```python
from build123d import *

# Parameters (mm, degrees)
SKETCH1_W           = 50
SKETCH1_H           = 200
BOSS_EXTRUDE1_DEPTH = 15
BOSS_EXTRUDE2_DEPTH = 20
BOSS_EXTRUDE3_DEPTH = 15


with BuildPart() as part:
    # Sketch1 → Boss-Extrude1 (new body)
    with BuildSketch(Plane(origin=(0, 0, 0), x_dir=(1, 0, 0), z_dir=(0, 1, 0))):
        Rectangle(SKETCH1_W, SKETCH1_H)
    extrude(amount=BOSS_EXTRUDE1_DEPTH)

    # Sketch2 → Boss-Extrude2 (add)
    with BuildSketch(Plane(origin=(0, 0, -30), x_dir=(-1, 0, 0), z_dir=(0, 0, -1))):
        with BuildLine():
            Line((25, 15), (25, 265))
            Line((25, 265), (-225, 265))
            Line((-225, 265), (-225, 215))
            ThreePointArc((-225, 215), (-82.144079422, 157.855920578), (-25, 15))
            Line((-25, 15), (25, 15))
        make_face()
        with BuildLine():
            Line((-25, 228.25), (-175, 228.25))
            ThreePointArc((-175, 228.25), (-186.75, 240), (-175, 251.75))
            Line((-175, 251.75), (-25, 251.75))
            ThreePointArc((-25, 251.75), (-13.25, 240), (-25, 228.25))
        make_face(mode=Mode.SUBTRACT)
    extrude(amount=BOSS_EXTRUDE2_DEPTH)

    # Sketch4 → Boss-Extrude3 (add)
    with BuildSketch(Plane.ZY.offset(7.5)):
        Polygon((-30, 115), (70, 15), (-30, 15), align=None)
    extrude(amount=-BOSS_EXTRUDE3_DEPTH)


solid = part.part
```
The model under review builds one solid part; all positions refer to its coordinate system, in mm. A direction names the side the tool comes from. Round coordinates to 2 decimals unless told otherwise and drop trailing zeros. Loops run counter-clockwise (first coordinate to the right, second up) from the corner with the lowest first, then second, coordinate; pieces in that order, holes last.
Item 1: Take a section at C-C (z = 38). Write out the cut boundary in (x, y).
Determined:
outline: (-25, 0) - (25, 0) - (25, 15) - (7.5, 15) - (7.5, 47) - (-7.5, 47) - (-7.5, 15) - (-25, 15) - close
Item 2: Clearance check with flat-ended pins moving along their axes: pin 1 Ø10 at (x, y) = (58.5, 198) entering from -Z; pin 2 Ø12 at (x, y) = (57, 127.5) entering from +Z; pin 3 Ø15 at (x, z) = (-12.5, 51.5) entering from +Y. State where each tip first meets the part, or that it passes through.
Determined:
pin 1: stops at z = -50
pin 2: stops at z = -30
pin 3: stops at y = 39.09
Item 3: For faces 4 (the face through (-11, 15, 34)), 5 (the face through (7.5, 43, -2)), 6 (the face through (74, 170, -50)), 7 (the face through (13.253, 240.258, -39.86)), list the 3-axis set-ups (+Z, -Z, +X, -X, +Y, -Y) from which the entire face can be reached by the end or side of a thin tool; tool diameter is ignored.
Determined:
face 4: +Z, +Y
face 5: +Z, +X, +Y
face 6: -Z, +X, -X, +Y
face 7: +Z, -Z
Item 4: Take a section at A-A (y = 240). Write out the cut boundary in (x, z), then the cut area to 3 significant figures.
Determined:
outline: (-25, -50) - (13.25, -50) - (13.25, -30) - (-25, -30) - close; (186.75, -50) - (225, -50) - (225, -30) - (186.75, -30) - close
area: 1,530 mm2
Item 5: Take a section at B-B (x = 126.5). Write out the cut boundary in (y, z).
Determined:
outline: (191.09, -50) - (228.25, -50) - (228.25, -30) - (191.09, -30) - close; (251.75, -50) - (265, -50) - (265, -30) - (251.75, -30) - close
Item 6: For line 1 (Z direction, x = 5.5, y = 137.5); line 2 (Y direction, x = 93.5, z = -37.5); line 3 (X direction, y = 31, z = 13.5), list the stretches that pass through material, from the lowest coordinate up.
Determined:
line 1: z = -50 to -30
line 2: y = 168.35 to 228.25, 251.75 to 265
line 3: x = -7.5 to 7.5
Item 7: Mouldability with a two-part tool opening along Y and no side actions: class faces 1 (the face through (0, 15, -75)), 2 (the face through (225, 240, -40)), 3 (the face through (101, 251.75, -40)) as released by +Y, released by -Y, zero draft, split by the parting line, or undercut.
Determined:
face 1: released by +Y
face 2: zero draft
face 3: undercut
Item 8: Take a section at D-D (y = 57). Write out the cut boundary in (x, z), then the cut area to 3 significant figures.
Determined:
outline: (-25, -50) - (28.53, -50) - (28.53, -30) - (7.5, -30) - (7.5, 28) - (-7.5, 28) - (-7.5, -30) - (-25, -30) - close
area: 1,940 mm2
